from build123d import *

# Parameters (mm, degrees)
F0_R     = 8
F0_W     = 20
F0_H     = 2
F1_DEPTH = 5


with BuildPart() as f1:
    # F0 (on Top) → F1 (new body)
    with BuildSketch(Plane.XY):
        Polygon((28.224968, -25.266338), (17.812495, -25.266338), (17.812495, -35.266338), (17.812495, -45.266338), (31.812495, -45.266338), (31.812495, -57.266338), (32.812495, -57.266338), (52.812495, -57.266338), (53.812495, -57.266338), (53.812495, -45.266338), (67.812495, -45.266338), (67.812495, -25.266338), (57.400022, -25.266338), align=None)
        with Locations((29.812495, -35.266338)):
            Circle(F0_R, mode=Mode.SUBTRACT)
        with BuildLine():
            ThreePointArc((44.317, -51.059522), (42.812495, -51.469457), (41.30799, -51.059522))
            ThreePointArc((41.30799, -51.059522), (42.812495, -50.649587), (44.317, -51.059522))
        make_face(mode=Mode.SUBTRACT)
        with BuildLine():
            ThreePointArc((42.812495, -41.474152), (43.744123, -45.047218), (42.812495, -48.620284))
            ThreePointArc((42.812495, -48.620284), (41.880867, -45.047218), (42.812495, -41.474152))
        make_face(mode=Mode.SUBTRACT)
        with Locations((55.812495, -35.266338)):
            Circle(F0_R, mode=Mode.SUBTRACT)
        Polygon((13.637441, 0), (28.224968, -25.266338), (57.400022, -25.266338), (71.987549, 0), (57.400022, 25.266338), (42.812495, 0), (28.224968, 25.266338), align=None)
        with Locations((42.812495, -58.266338)):
            Rectangle(F0_W, F0_H)
    extrude(amount=F1_DEPTH)


solid = f1.part
Build history of the part. All positions in model axes, mm. A direction names the side the tool comes from. Coordinates: 2 decimals unless noted, no trailing zeros. Order: outer loops, then holes, each group sorted by start corner. A loop starts at its lowest first (then second) coordinate and runs counter-clockwise, first axis right, second up. Notation, with made-up numbers: (-35, 38) - (-1, 38) arc R28 ccw to (-1, 66) - close; hole circle Ø8 at (82, 18.25). An arc over 180 degrees is marked (long way). Write each question's results on one line, items separated by ' | '. Start each with the question number.
Item 1: Band-saw the part on B-B on x = 51. Write the cut outline in (y, z), and give its area (3 significant figures).
Item 2: Band-saw the part on C-C on z = 2.2. Write the cut outline in (x, y), and give its area (3 significant figures).
Item 3: Tool access for faces 5 (the face through (25, -45.266, 2)), 6 (the face through (23, -25.266, 2)), 7 (the face through (53.812, -51, 2)): list every direction of +Z, -Z, +X, -X, +Y, -Y with a clear straight run to the whole face (end or side of a thin tool).
Item 4: Band-saw the part on D-D on y = -21. Write the cut outline in (x, z), and give its area (3 significant figures).
Item 5: Mould opens along Y. For faces 1 (the face through (32.812, -58, 2)), 2 (the face through (64.59, -12.81, 2.46)), 3 (the face through (61, -45.266, 2)), 4 (the face through (41.88, -45.1, 2.46)) say: released by +Y, released by -Y, zero draft, split by the parting line, or undercut.
Item 6: Flat gauge pins, fed straight in: pin 1 (0.5 mm diameter, centred on x = 32.5, z = 1.5, fed in from -Y); pin 2 (1.5 mm diameter, centred on x = 49.5, z = 1, fed in from +Y); pin 3 (1.5 mm diameter, centred on y = -48.5, z = 0.5, fed in from +X); pin 4 (14.5 mm diameter, centred on x = 29.81, y = -35.27, fed in from +Z). Where does each tip first touch, or does it go through?
Item 7: Wall check: probe 1 along Y at (x, z) = (63, 0.5); probe 2 along X at (y, z) = (4.5, 0.55); probe 3 along Y at (x, z) = (33, 4). Give the ranges that are in metal, low to high. Write a range as [from, to].
Item 8: Band-saw the part on A-A on y = 13.5. Write the cut outline in (x, z), and give its area (3 significant figures).
Numbers:
1) outline: (-59.27, 0) - (-41.66, 0) - (-41.66, 5) - (-59.27, 5) - close; (-28.88, 0) - (14.18, 0) - (14.18, 5) - (-28.88, 5) - close | area: 303 mm^2
2) outline: (13.64, 0) - (28.22, -25.27) - (17.81, -25.27) - (17.81, -45.27) - (31.81, -45.27) - (31.81, -57.27) - (32.81, -57.27) - (32.81, -59.27) - (52.81, -59.27) - (52.81, -57.27) - (53.81, -57.27) - (53.81, -45.27) - (67.81, -45.27) - (67.81, -25.27) - (57.4, -25.27) - (71.99, 0) - (57.4, 25.27) - (42.81, 0) - (28.22, 25.27) - close; hole circle Ø16 at (29.81, -35.27); hole (41.31, -51.06) arc R2.97 ccw to (44.32, -51.06) arc R2.97 ccw to start; hole (42.81, -48.62) arc R7.32 ccw to (42.81, -41.47) arc R7.32 ccw to start; hole circle Ø16 at (55.81, -35.27) | area: 2,730 mm^2
3) face 5: +Z, -Z, -X, -Y | face 6: +Z, -Z, -X | face 7: +Z, -Z, +X, -Y
4) outline: (25.76, 0) - (59.86, 0) - (59.86, 5) - (25.76, 5) - close | area: 171 mm^2
5) face 1: zero draft | face 2: undercut | face 3: released by -Y | face 4: undercut
6) pin 1: y = -57.27 | pin 2: y = 12.88 | pin 3: x = 53.81 | pin 4: through
7) probe 1: [-45.27, -38.78], [-31.75, -25.27], [-15.57, 15.57] | probe 2: [16.24, 40.21], [45.41, 69.39] | probe 3: [-59.27, -42.6], [-27.93, 17]
8) outline: (21.43, 0) - (35.02, 0) - (35.02, 5) - (21.43, 5) - close; (50.61, 0) - (64.19, 0) - (64.19, 5) - (50.61, 5) - close | area: 136 mm^2
